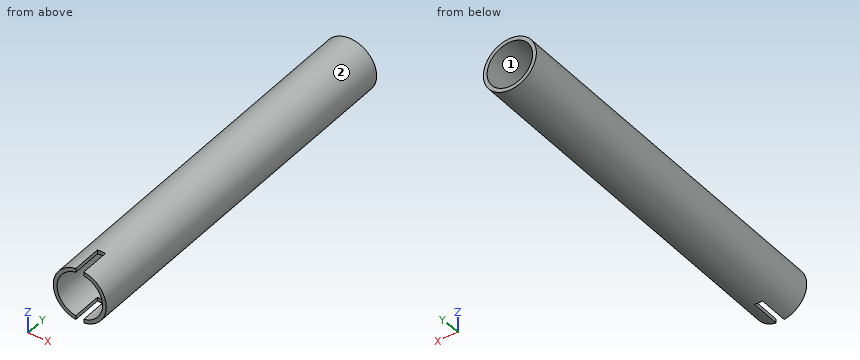
```python
from build123d import *

# Parameters (mm, degrees)
F0_R     = 44.45
F0_R_2   = 38.1
F1_DEPTH = 317.5
F2_W     = 13.335
F2_H     = 50.8
F3_DEPTH = 44.451
F4_DEPTH = 44.451


with BuildPart() as f1:
    # F0 (on Front) → F1 (new body, symmetric)
    with BuildSketch(Plane.XZ):
        Circle(F0_R)
        Circle(F0_R_2, mode=Mode.SUBTRACT)
    extrude(amount=F1_DEPTH, both=True)

    # F2 (on Top) → F3 (cut, through all)
    with BuildSketch(Plane.XY):
        with Locations((0, -342.9)):
            Rectangle(F2_W, F2_H)
        with Locations((0, -292.1)):
            Rectangle(F2_W, F2_H)
    extrude(amount=F3_DEPTH, mode=Mode.SUBTRACT)

    # F2 (on Top) → F4 (cut, through all)
    with BuildSketch(Plane.XY):
        with Locations((0, -292.1)):
            Rectangle(F2_W, F2_H)
    extrude(amount=-F4_DEPTH, mode=Mode.SUBTRACT)


solid = f1.part
```
The listing builds one solid part. Answer for the finished solid, in the listing's coordinates (mm). Face numbers are marked on the shaded views. Give positions to 0.01 mm unless a question says otherwise; leave off trailing zeros. Order: outer loops, then holes, each group sorted by start corner. A loop starts at its lowest first (then second) coordinate and runs counter-clockwise, first axis right, second up. Notation, with made-up numbers: (-21, 38.5) -> (0, 38.5) arc R17 cw to (0, 42.5) -> close; hole circle Ø4 at (1.25, 86.25). An arc over 180 degrees is marked (long way). Answer as a JSON object with one key per item and string values. Group by question number.
Item 1: Determine the mould class of the marked faces 1 and 2 for opening direction X: pulls with the +X half, pulls with the -X half, needs draft (parallel to the pull), parting line crosses it, or undercut.
Item 2: Flat-ended cylindrical pins translate along their axes: pin 1 (2 mm diameter, centred on y = -211.5, z = -27, fed in from +X); pin 2 (1.9 mm diameter, centred on y = -285.5, z = 39.5, fed in from +X); pin 3 (4 mm diameter, centred on x = -3.5, y = 223.5, fed in from +Z). Find the tip coordinate at first contact, or state that the pin passes through.
Item 3: The part is cut by section C-C on y = 232. Write down the section's boundary in (x, z), and give its area (3 significant figures).
Item 4: The part is cut by section A-A on x = 0. Write down the section's boundary in (y, z).
Item 5: The part is cut by section B-B on z = 0. Write down the section's boundary in (x, y), and give its area (3 significant figures).
Item 6: Consider L1, parallel to X at y = 50.5, z = 0; L2, parallel to Z at x = -1, y = 105; L3, parallel to Z at x = -10, y = -249. Determine where each line is inside the solid, lowest interval first. Write a range as from..to.
Result set:
{
 "1": {"face 1": "undercut", "face 2": "parting line crosses it"},
 "2": {"pin 1": "x = 36.05", "pin 2": "x = 22.13", "pin 3": "z = 44.42"},
 "3": {"outline": "circle Ø88.9 at (0, 0); hole circle Ø76.2 at (0, 0)", "area": "1,650 mm²"},
 "4": {"outline": "(-266.7, -44.45) -> (317.5, -44.45) -> (317.5, -38.1) -> (-266.7, -38.1) -> close; (-266.7, 38.1) -> (317.5, 38.1) -> (317.5, 44.45) -> (-266.7, 44.45) -> close"},
 "5": {"outline": "(-44.45, -317.5) -> (-38.1, -317.5) -> (-38.1, 317.5) -> (-44.45, 317.5) -> close; (38.1, -317.5) -> (44.45, -317.5) -> (44.45, 317.5) -> (38.1, 317.5) -> close", "area": "8,060 mm²"},
 "6": {"L1": "-44.45..-38.1, 38.1..44.45", "L2": "-44.44..-38.09, 38.09..44.44", "L3": "-43.31..-36.76, 36.76..43.31"}
}
